```python
from build123d import *

# Parameters (mm, degrees)
SKETCH_R     = 8
PAD_DEPTH    = 200
SKETCH001_R  = 7.5
POCKET_DEPTH = 200
PAD001_DEPTH = 200


with BuildPart() as part:
    # Sketch → Pad (new body)
    with BuildSketch(Plane.XY):
        Circle(SKETCH_R)
    extrude(amount=PAD_DEPTH)

    # Sketch001 (on Face3 of Pad) → Pocket (cut)
    with BuildSketch(Plane.XY.offset(200)):
        Circle(SKETCH001_R)
    extrude(amount=-POCKET_DEPTH, mode=Mode.SUBTRACT)

    # Sketch002 (on Face3 of Pocket) → Pad001 (join)
    with BuildSketch(Plane.XY.offset(200)):
        Polygon((-0.25, 7.75), (0.25, 7.75), (0.25, 0.25), (7.75, 0.25), (7.75, -0.25), (0.25, -0.25), (0.25, -7.75), (-0.25, -7.75), (-0.25, -0.25), (-7.75, -0.25), (-7.75, 0.25), (-0.25, 0.25), align=None)
    extrude(amount=-PAD001_DEPTH)


solid = part.part
```
Design review of the part built by this model. Coordinates are the model's own, in mm. A direction names the side the tool comes from. Coordinates: 2 decimals unless noted, no trailing zeros. Write each loop counter-clockwise with the first axis right and the second up, starting at its lowest first coordinate (ties: lowest second). Pieces come first, ordered by that corner, then holes. Notation, with made-up numbers: M 86.25,51.5 L 135.25,51.5 A29 cw 135.25,72.5 Z; hole C 38.5,60.25 d4. An arc over 180 degrees is marked long. Answer as a JSON object with one key per item and string values.
Item 1: Wall thickness on probe 1 along Y at (x, z) = (0.75, 191); probe 2 along X at (y, z) = (1.5, 173); probe 3 along Y at (x, z) = (-6.5, 123): over which ranges is each line inside the solid? List them lowest first.
Outcome:
{"probe 1": "-7.96 to -7.46, -0.25 to 0.25, 7.46 to 7.96", "probe 2": "-7.86 to -7.35, -0.25 to 0.25, 7.35 to 7.86", "probe 3": "-4.66 to -3.74, -0.25 to 0.25, 3.74 to 4.66"}
Item 2: Insertion check: pin 1 Ø8 at (x, z) = (3.5, 140.5) entering from -Y; pin 2 Ø6 at (x, z) = (6, 82) entering from -Y; pin 3 Ø1.5 at (y, z) = (3.5, 147) entering from +X; pin 4 Ø8 at (y, z) = (4.5, 56.5) entering from -X. Each pin has a flat end and moves straight along its axis. Give the tip position at first contact, or say it passes through.
Outcome:
{"pin 1": "y = -8", "pin 2": "y = -7.42", "pin 3": "x = 7.51", "pin 4": "x = -7.98"}
Item 3: Add section B-B, the plane y = 4. Give the boundary of the cut face in (x, z).
Outcome:
{"outline": "M -6.93,0 L -6.34,0 L -6.34,200 L -6.93,200 Z; M -0.25,0 L 0.25,0 L 0.25,200 L -0.25,200 Z; M 6.34,0 L 6.93,0 L 6.93,200 L 6.34,200 Z"}
Item 4: Add section C-C, the plane x = -2.75. Give the boundary of the cut face in (y, z), and give its area (3 significant figures).
Outcome:
{"outline": "M -7.51,0 L -6.98,0 L -6.98,200 L -7.51,200 Z; M -0.25,0 L 0.25,0 L 0.25,200 L -0.25,200 Z; M 6.98,0 L 7.51,0 L 7.51,200 L 6.98,200 Z", "area": "314 mm²"}
Item 5: Add section A-A, the plane z = 84. Give the boundary of the cut face in (x, y), and give its area (3 significant figures).
Outcome:
{"outline": "C 0,0 d16; hole M -7.5,-0.25 A7.5 ccw -0.25,-7.5 L -0.25,-0.25 Z; hole M -7.5,0.25 L -0.25,0.25 L -0.25,7.5 A7.5 ccw Z; hole M 0.25,-7.5 A7.5 ccw 7.5,-0.25 L 0.25,-0.25 Z; hole M 0.25,0.25 L 7.5,0.25 A7.5 ccw 0.25,7.5 Z", "area": "39.1 mm²"}
Item 6: Machinability: for faces 4 (the cylindrical face through (-5.359, -5.247, 101.4)), 5 (the flat face through (0, -1, 200)), which of the approach directions +Z, -Z, +X, -X, +Y, -Y give a long, thin tool a straight path to every point of the face, cutting with its end or side? Answer none if there is none.
Outcome:
{"face 4": "+Z, -Z", "face 5": "+Z, +X, -X, +Y, -Y"}
Item 7: Draft analysis for pull direction Y (two halves, no side actions). For faces 1 (the cylindrical face through (-1.73, -7.81, 98.6)), 2 (the flat face through (0, -1, 0)), 3 (the flat face through (-4, -0.25, 101)), state which applies: pulls with the +Y half, pulls with the -Y half, needs draft (parallel to the pull), parting line crosses it, or undercut.
Outcome:
{"face 1": "parting line crosses it", "face 2": "needs draft", "face 3": "undercut"}
